Design review of the part built by this model. Coordinates are the model's own, in mm. A direction names the side the tool comes from. Round coordinates to 2 decimals unless told otherwise and drop trailing zeros. Order: outer loops, then holes, each group sorted by start corner. A loop starts at its lowest first (then second) coordinate and runs counter-clockwise, first axis right, second up.
from build123d import *

# Parameters (mm, degrees)
SKETCH1_W           = 20
SKETCH1_H           = 105
SKETCH1_R           = 1.55
SKETCH1_H_2         = 15
SKETCH1_R_2         = 1.5
SKETCH1_W_2         = 28
SKETCH1_R_3         = 4
BOSS_EXTRUDE1_DEPTH = 2
FILLET1_R           = 6


with BuildPart() as part:
    # Sketch1 → Boss-Extrude1 (new, symmetric)
    # profile 1 of 3: a face of its own
    with BuildSketch(Plane.XY):
        with Locations((-14, 60)):
            Rectangle(SKETCH1_W, SKETCH1_H)
        with Locations((-14, 27.1)):
            Circle(SKETCH1_R, mode=Mode.SUBTRACT)
        with Locations((-14, 87.1)):
            Circle(SKETCH1_R, mode=Mode.SUBTRACT)
    # profile 2 of 3: a face of its own
    with BuildSketch(Plane.XY):
        with Locations((-14, 0)):
            Rectangle(SKETCH1_W, SKETCH1_H_2)
        with Locations((-18, 0)):
            Circle(SKETCH1_R_2, mode=Mode.SUBTRACT)
    # profile 3 of 3: a face of its own
    with BuildSketch(Plane.XY):
        with Locations((10, 0)):
            Rectangle(SKETCH1_W_2, SKETCH1_H_2)
        with Locations((14, 0)):
            Circle(SKETCH1_R_3, mode=Mode.SUBTRACT)
    extrude(amount=BOSS_EXTRUDE1_DEPTH, both=True)

    # Fillet1
    fillet1_edges = [part.edges().sort_by_distance(p)[0] for p in [
        (-24, 112.5, 0),
        (-4, 112.5, 0),
        (-4, 7.5, 0),
        (24, 7.5, 0),
        (24, -7.5, 0),
        (-24, -7.5, 0),
    ]]
    fillet(fillet1_edges, radius=FILLET1_R)


solid = part.part
1) For faces 4 (the face through (0, -7.5, 0)), 5 (the face through (-4, 59, 0)), list the 3-axis set-ups (+Z, -Z, +X, -X, +Y, -Y) from which the entire face can be reached by the end or side of a thin tool; tool diameter is ignored.
Results:
face 4: +Z, -Z, +X, -X, -Y
face 5: +Z, -Z, +X, +Y
2) Take a section at B-B on y = 27.1. Give the boundary of the cut face in (x, z), plus the area to 3 significant figures.
Results:
outline: (-24, -2) - (-15.55, -2) - (-15.55, 2) - (-24, 2) - close; (-12.45, -2) - (-4, -2) - (-4, 2) - (-12.45, 2) - close
area: 67.6 mm2
3) Take a section at D-D on x = 4. Give the boundary of the cut face in (y, z), plus the area to 3 significant figures.
Results:
outline: (-7.5, -2) - (7.5, -2) - (7.5, 2) - (-7.5, 2) - close
area: 60.0 mm2
4) Take a section at C-C on z = -1.1. Give the boundary of the cut face in (x, y), plus the area to 3 significant figures.
Results:
outline: (-24, -1.5) arc R6 ccw to (-18, -7.5) - (18, -7.5) arc R6 ccw to (24, -1.5) - (24, 1.5) arc R6 ccw to (18, 7.5) - (2, 7.5) arc R6 cw to (-4, 13.5) - (-4, 106.5) arc R6 ccw to (-10, 112.5) - (-18, 112.5) arc R6 ccw to (-24, 106.5) - close; hole circle Ø3 at (-18, 0); hole circle Ø3.1 at (-14, 27.1); hole circle Ø3.1 at (-14, 87.1); hole circle Ø8 at (14, 0)
area: 2,720 mm2
5) Take a section at A-A on x = -14. Give the boundary of the cut face in (y, z).
Results:
outline: (-7.5, -2) - (25.55, -2) - (25.55, 2) - (-7.5, 2) - close; (28.65, -2) - (85.55, -2) - (85.55, 2) - (28.65, 2) - close; (88.65, -2) - (112.5, -2) - (112.5, 2) - (88.65, 2) - close
6) The part is to be moulded in two halves that separate along X. For faces 1 (the face through (-14, 112.5, 0)), 2 (the face through (10, 0, 0)), 3 (the face through (22.196, 5.789, 0.028)), say which applies: released by +X, released by -X, zero draft, split by the parting line, or undercut.
Results:
face 1: zero draft
face 2: undercut
face 3: released by +X
7) Clearance check with flat-ended pins moving along their axes: P1, Ø2, axis at y = 55.5, z = 1, coming from the +X side; P2, Ø1.2, axis at x = 7.5, z = -1, coming from the +Y side. State where each tip first meets the part, or that it passes through.
Results:
P1: stops at x = -4
P2: stops at y = 7.5
8) To check wall thickness, follow line 1 along Y through (x, z) = (-14, -0.9); line 2 along X through (y, z) = (87.1, 0.2); line 3 along Y through (x, z) = (-18, 0.3). State the ranges of each line that lie inside material, in increasing order.
Results:
line 1: y = -7.5 to 25.55, 28.65 to 85.55, 88.65 to 112.5
line 2: x = -24 to -15.55, -12.45 to -4
line 3: y = -7.5 to -1.5, 1.5 to 112.5
